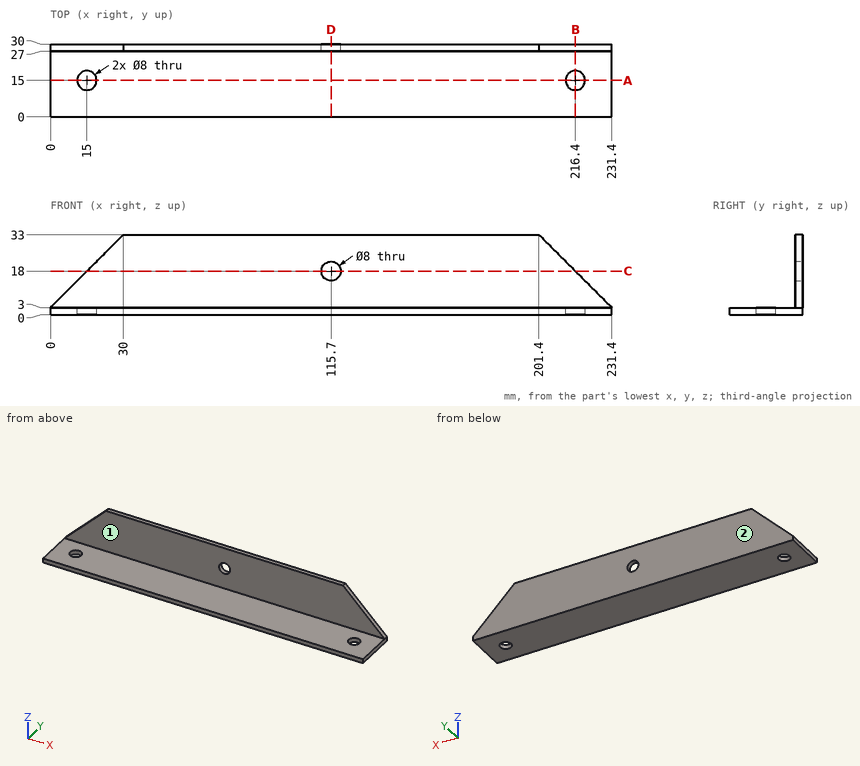
Answer from the drawing. Dimensions are ordinates in mm from the lowest x, y and z of the part. A direction names the side the tool comes from. Give positions to 0.01 mm unless a question says otherwise; leave off trailing zeros. Order: outer loops, then holes, each group sorted by start corner. A loop starts at its lowest first (then second) coordinate and runs counter-clockwise, first axis right, second up.
(1) Find section B-B (x = 216.4). Give the vertices of the cut face in (y, z).
(2) For the marked faces 1 and 2, determine the directions among +Z, -Z, +X, -X, +Y, -Y from which every point of the face is accessible in a straight line to the end or side of a thin tool.
(3) Find section D-D (x = 115.7). Give the vertices of the cut face in (y, z).
(4) Straight lines are drawn through the part: L1, parallel to Z at x = 115.7, y = 28.3; L2, parallel to Z at x = 118, y = 26.75; L3, parallel to Y at x = 34.5, z = 24. For each, find the intervals that lie inside material, in ascending order.
(5) Find section A-A (y = 15). Give the vertices of the cut face in (x, z), plus the area to 3 significant figures.
(6) Find section C-C (z = 18). Give the vertices of the cut face in (x, y), plus the area to 3 significant figures.
(7) Given pin 1 (8 mm diameter, centred on x = 46.5, y = 11.5, fed in from +Z), flat-ended and moving along its own axis, determine where the tip first touches the part or whether it passes through.
Result sheet:
1. outline: (0, 0) - (11, 0) - (11, 3) - (0, 3) - close; (19, 0) - (30, 0) - (30, 18) - (27, 18) - (27, 3) - (19, 3) - close
2. face 1: +Z, +X, -X, -Y
2. face 2: +Z, -Z, +X, -X, +Y
3. outline: (0, 0) - (30, 0) - (30, 14) - (27, 14) - (27, 3) - (0, 3) - close; (27, 22) - (30, 22) - (30, 33) - (27, 33) - close
4. L1: z = 0 to 14, 22 to 33
4. L2: z = 0 to 3
4. L3: y = 27 to 30
5. outline: (0, 0) - (11, 0) - (11, 3) - (0, 3) - close; (19, 0) - (212.4, 0) - (212.4, 3) - (19, 3) - close; (220.4, 0) - (231.4, 0) - (231.4, 3) - (220.4, 3) - close
5. area: 646 mm2
6. outline: (15, 27) - (111.7, 27) - (111.7, 30) - (15, 30) - close; (119.7, 27) - (216.4, 27) - (216.4, 30) - (119.7, 30) - close
6. area: 580 mm2
7. pin 1: stops at z = 3
